Read the model definition and answer for the solid it produces. Units are mm, in the model's axes. Face numbers are marked on the shaded views. A direction names the side the tool comes from. Coordinates: 2 decimals unless noted, no trailing zeros. Write each loop counter-clockwise with the first axis right and the second up, starting at its lowest first coordinate (ties: lowest second). Pieces come first, ordered by that corner, then holes.
1) Each of these flat-tipped pins is pushed along its axis until it touches: pin 1 Ø0.8 at (x, z) = (-8.5, 1) entering from +Y; pin 2 Ø1.2 at (x, z) = (9, 1.5) entering from -Y; pin 3 Ø0.8 at (y, z) = (9, 1) entering from +X. Where does it stop, or does it pass through?
2) The part is cut by section D-D (y = 4.25). Determine the outline of the cut face in (x, z), then the cut area to 3 significant figures.
3) Determine the mould class of the marked faces 1, 2 and 3 for opening direction X: +X half, -X half, draft (parallel to the pull), parting line (faces both ways), or undercut.
4) The part is cut by section B-B (z = 0.4). Determine the outline of the cut face in (x, y) (3 decimals).
5) Find the intervals of material crossed by line 1 (Y direction, x = 0, z = 1.4) (3 decimals); line 2 (X direction, y = 0.25, z = 1); line 3 (Y direction, x = 3, z = 1.6), in increasing order.
6) Which of the six approach directions +Z, -Z, +X, -X, +Y, -Y give full straight-line access (tool end or side, diameter ignored) to the marked faces 4 and 5?
7) The part is cut by section C-C (x = -0.25). Determine the outline of the cut face in (y, z), then the cut area to 3 significant figures.
8) The part is cut by section A-A (y = 0). Determine the outline of the cut face in (x, z) (3 decimals).
from build123d import *

# Parameters (mm, degrees)
F0_R     = 12.5
F0_R_2   = 4.875
F1_DEPTH = 2


with BuildPart() as f1:
    # F0 (on Top) → F1 (new body)
    with BuildSketch(Plane.XY):
        Circle(F0_R)
        with BuildLine():
            ThreePointArc((-1.575, -8), (0, -6.425), (1.575, -8))
            Line((1.575, -8), (1.575, -9.5))
            ThreePointArc((1.575, -9.5), (0, -11.075), (-1.575, -9.5))
            Line((-1.575, -9.5), (-1.575, -8))
        make_face(mode=Mode.SUBTRACT)
        with BuildLine():
            ThreePointArc((-9.5, -1.575), (-11.075, 0), (-9.5, 1.575))
            Line((-9.5, 1.575), (-8, 1.575))
            ThreePointArc((-8, 1.575), (-6.425, 0), (-8, -1.575))
            Line((-8, -1.575), (-9.5, -1.575))
        make_face(mode=Mode.SUBTRACT)
        Circle(F0_R_2, mode=Mode.SUBTRACT)
        with BuildLine():
            Line((9.5, -1.575), (8, -1.575))
            ThreePointArc((8, -1.575), (6.425, 0), (8, 1.575))
            Line((8, 1.575), (9.5, 1.575))
            ThreePointArc((9.5, 1.575), (11.075, 0), (9.5, -1.575))
        make_face(mode=Mode.SUBTRACT)
        with BuildLine():
            Line((1.575, 9.5), (1.575, 8))
            ThreePointArc((1.575, 8), (0, 6.425), (-1.575, 8))
            Line((-1.575, 8), (-1.575, 9.5))
            ThreePointArc((-1.575, 9.5), (0, 11.075), (1.575, 9.5))
        make_face(mode=Mode.SUBTRACT)
    extrude(amount=F1_DEPTH)


solid = f1.part
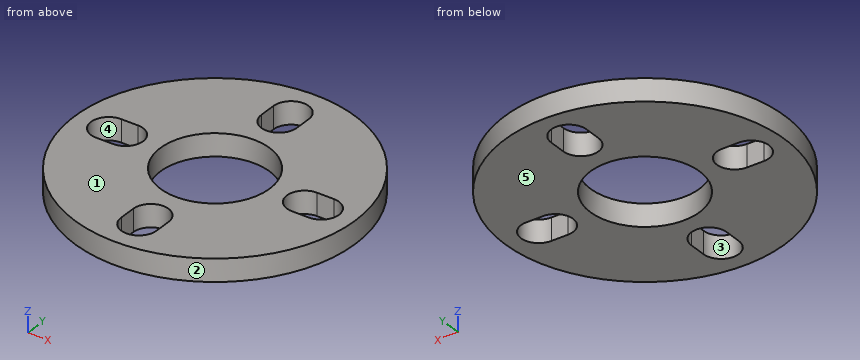
Reported:
1. pin 1: stops at y = 9.52
1. pin 2: stops at y = -9.26
1. pin 3: stops at x = 9.07
2. outline: (-11.76, 0) - (-2.39, 0) - (-2.39, 2) - (-11.76, 2) - close; (2.39, 0) - (11.76, 0) - (11.76, 2) - (2.39, 2) - close
2. area: 37.5 mm2
3. face 1: draft
3. face 2: parting line
3. face 3: undercut
4. outline: circle Ø25 at (0, 0); hole (-9.5, -1.575) - (-8, -1.575) arc R1.575 ccw to (-8, 1.575) - (-9.5, 1.575) arc R1.575 ccw to start; hole circle Ø9.75 at (0, 0); hole (-1.575, -9.5) arc R1.575 ccw to (1.575, -9.5) - (1.575, -8) arc R1.575 ccw to (-1.575, -8) - close; hole (-1.575, 8) arc R1.575 ccw to (1.575, 8) - (1.575, 9.5) arc R1.575 ccw to (-1.575, 9.5) - close; hole (8, -1.575) - (9.5, -1.575) arc R1.575 ccw to (9.5, 1.575) - (8, 1.575) arc R1.575 ccw to start
5. line 1: y = -12.5 to -11.075, -6.425 to -4.875, 4.875 to 6.425, 11.075 to 12.5
5. line 2: x = -12.5 to -11.06, -6.44 to -4.87, 4.87 to 6.44, 11.06 to 12.5
5. line 3: y = -12.13 to -3.84, 3.84 to 12.13
6. face 4: +Z, -Z
6. face 5: -Z, +X, -X, +Y, -Y
7. outline: (-12.5, 0) - (-11.06, 0) - (-11.06, 2) - (-12.5, 2) - close; (-6.44, 0) - (-4.87, 0) - (-4.87, 2) - (-6.44, 2) - close; (4.87, 0) - (6.44, 0) - (6.44, 2) - (4.87, 2) - close; (11.06, 0) - (12.5, 0) - (12.5, 2) - (11.06, 2) - close
7. area: 12.1 mm2
8. outline: (-12.5, 0) - (-11.075, 0) - (-11.075, 2) - (-12.5, 2) - close; (-6.425, 0) - (-4.875, 0) - (-4.875, 2) - (-6.425, 2) - close; (4.875, 0) - (6.425, 0) - (6.425, 2) - (4.875, 2) - close; (11.075, 0) - (12.5, 0) - (12.5, 2) - (11.075, 2) - close
